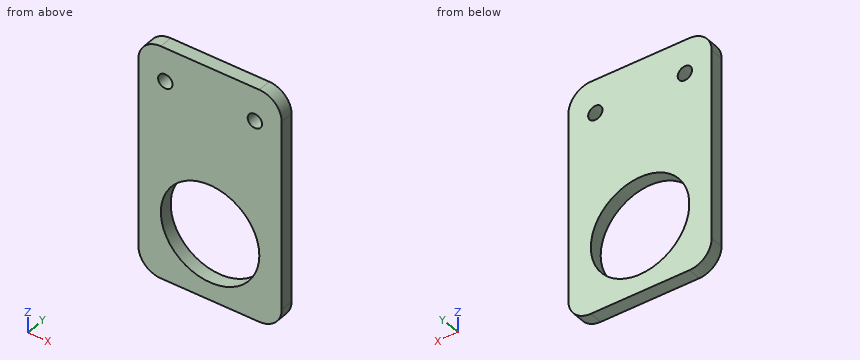
```python
from build123d import *

# Parameters (mm, degrees)
SKETCH1_W           = 32
SKETCH1_H           = 52.5
SKETCH1_R           = 11
SKETCH1_R_2         = 1.6
BOSS_EXTRUDE1_DEPTH = 3
FILLET1_R           = 5


with BuildPart() as part:
    # Sketch1 → Boss-Extrude1 (new body)
    with BuildSketch(Plane(origin=(0, 0, 0), x_dir=(1, 0, 0), z_dir=(0, 1, 0))):
        with Locations((16, 26.25)):
            Rectangle(SKETCH1_W, SKETCH1_H)
        with Locations((16, 37.5)):
            Circle(SKETCH1_R, mode=Mode.SUBTRACT)
        with Locations((6, 7.5)):
            Circle(SKETCH1_R_2, mode=Mode.SUBTRACT)
        with Locations((26, 7.5)):
            Circle(SKETCH1_R_2, mode=Mode.SUBTRACT)
    extrude(amount=BOSS_EXTRUDE1_DEPTH)

    # Fillet1
    fillet1_edges = [part.edges().sort_by_distance(p)[0] for p in [
        (0, 1.5, -52.5),
        (32, 1.5, -52.5),
        (32, 1.5, 0),
        (0, 1.5, 0),
    ]]
    fillet(fillet1_edges, radius=FILLET1_R)


solid = part.part
```
Work out the finished part from the listing and answer in its coordinate system (mm). Coordinates: 2 decimals unless noted, no trailing zeros. Write each loop counter-clockwise with the first axis right and the second up, starting at its lowest first coordinate (ties: lowest second). Pieces come first, ordered by that corner, then holes. Notation, with made-up numbers: (-18, 67) - (40, 67) arc R22 ccw to (40, 84) - close; hole circle Ø9 at (-6, 31.5). An arc over 180 degrees is marked (long way). Answer as a JSON object with one key per item and string values.
Q1. Consider L1, parallel to X at y = 0.75, z = -7.5; L2, parallel to Z at x = 16, y = 1.9; L3, parallel to Z at x = 25, y = 2.05. Determine where each line is inside the solid, lowest interval first. Write a range as from..to.
Results list:
{"L1": "x = 0..4.4, 7.6..24.4, 27.6..32", "L2": "z = -52.5..-48.5, -26.5..0", "L3": "z = -52.5..-43.82, -31.18..-8.75, -6.25..0"}
Q2. Find section A-A (x = 16). Write down the section's boundary in (y, z), plus the area to 3 significant figures.
Results list:
{"outline": "(0, -52.5) - (3, -52.5) - (3, -48.5) - (0, -48.5) - close; (0, -26.5) - (3, -26.5) - (3, 0) - (0, 0) - close", "area": "91.5 mm^2"}
Q3. Given pin 1 Ø5 at (x, z) = (18, -9) entering from -Y, flat-ended and moving along its own axis, determine where the tip first touches the part or whether it passes through.
Results list:
{"pin 1": "stops at y = 0"}
Q4. Find section C-C (z = -7.5). Write down the section's boundary in (x, y).
Results list:
{"outline": "(0, 0) - (4.4, 0) - (4.4, 3) - (0, 3) - close; (7.6, 0) - (24.4, 0) - (24.4, 3) - (7.6, 3) - close; (27.6, 0) - (32, 0) - (32, 3) - (27.6, 3) - close"}
Q5. Find section D-D (z = -37.5). Write down the section's boundary in (x, y), plus the area to 3 significant figures.
Results list:
{"outline": "(0, 0) - (5, 0) - (5, 3) - (0, 3) - close; (27, 0) - (32, 0) - (32, 3) - (27, 3) - close", "area": "30.0 mm^2"}
Q6. Find section B-B (y = 2.2). Write down the section's boundary in (x, z).
Results list:
{"outline": "(0, -47.5) arc R5 ccw to (5, -52.5) - (27, -52.5) arc R5 ccw to (32, -47.5) - (32, -5) arc R5 ccw to (27, 0) - (5, 0) arc R5 ccw to (0, -5) - close; hole circle Ø3.2 at (6, -7.5); hole circle Ø22 at (16, -37.5); hole circle Ø3.2 at (26, -7.5)"}
